Can you work these out from the drawing? Everything is in mm from the part's minimum corner. A direction names the side the tool comes from. Coordinates: 2 decimals unless noted, no trailing zeros. Loops run counter-clockwise (first coordinate to the right, second up) from the corner with the lowest first, then second, coordinate; pieces in that order, holes last.
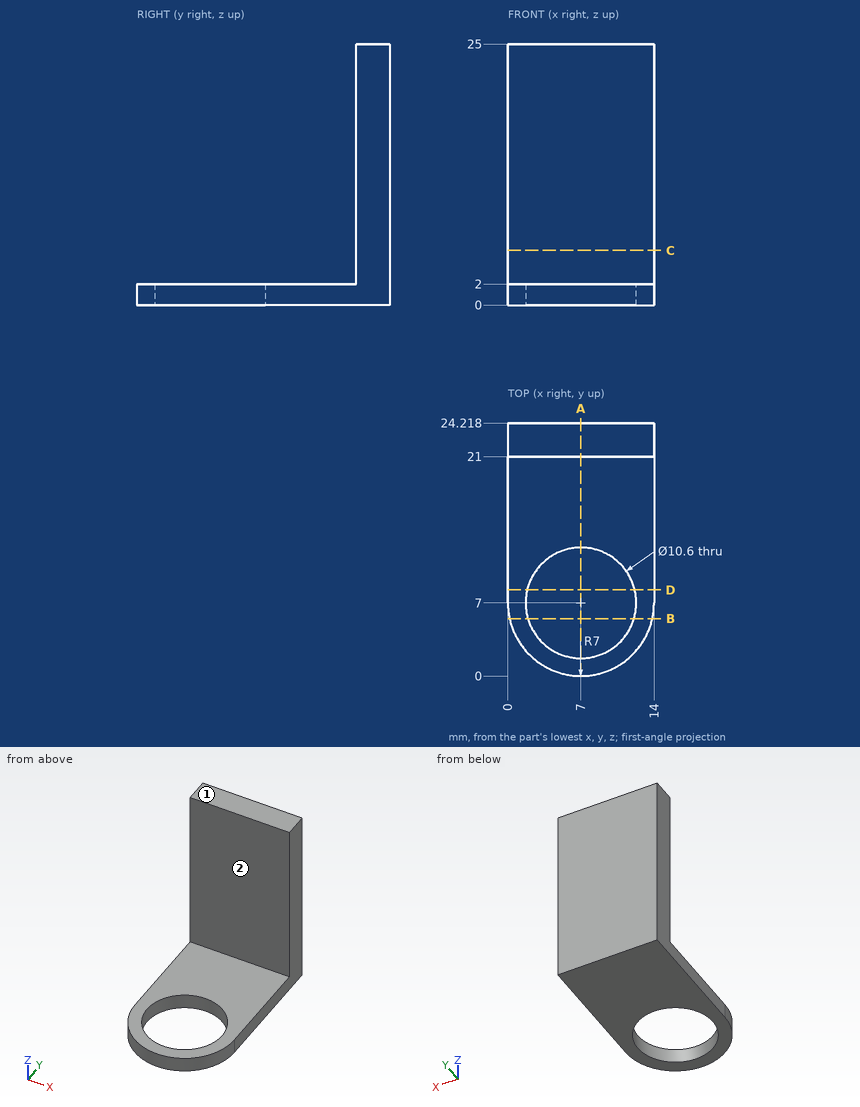
(1) Imagine slicing it at A-A, the plane x = 7. Write out the boundary of the cut face in (y, z), and give its area (3 significant figures).
Answers:
outline: (0, 0) - (1.7, 0) - (1.7, 2) - (0, 2) - close; (12.3, 0) - (24.22, 0) - (24.22, 25) - (21, 25) - (21, 2) - (12.3, 2) - close
area: 101 mm2
(2) Imagine slicing it at C-C, the plane z = 5.25. Write out the boundary of the cut face in (x, y).
Answers:
outline: (0, 21) - (14, 21) - (14, 24.22) - (0, 24.22) - close
(3) Which directions (+Z, -Z, +X, -X, +Y, -Y) give clear straight access to the entire face, cutting with the end or side of a thin tool? Please do the marked faces 1 and 2.
Answers:
face 1: +Z, +X, -X, +Y, -Y
face 2: +Z, +X, -X, -Y
(4) Imagine slicing it at B-B, the plane y = 5.5. Write out the boundary of the cut face in (x, z).
Answers:
outline: (0.16, 0) - (1.92, 0) - (1.92, 2) - (0.16, 2) - close; (12.08, 0) - (13.84, 0) - (13.84, 2) - (12.08, 2) - close
(5) Imagine slicing it at D-D, the plane y = 8.25. Write out the boundary of the cut face in (x, z).
Answers:
outline: (0, 0) - (1.85, 0) - (1.85, 2) - (0, 2) - close; (12.15, 0) - (14, 0) - (14, 2) - (12.15, 2) - close
(6) For pin 1 (4 mm diameter, centred on x = 9.5, y = 6, fed in from +Z); pin 2 (4 mm diameter, centred on x = 8, z = 19, fed in from -Y), each with a flat end and sliding along its axis, tell me the tip position at first contact or that it passes through.
Answers:
pin 1: passes through
pin 2: stops at y = 21
(7) I need wall thicknesses on probe 1 along Y at (x, z) = (7, 1.15); probe 2 along Z at (x, y) = (4.5, 12.5); probe 3 along Y at (x, z) = (8, 13.5). Which ranges of each line are inside material? Lowest first, please.
Answers:
probe 1: y = 0 to 1.7, 12.3 to 24.22
probe 2: z = 0 to 2
probe 3: y = 21 to 24.22
